Build history of the part. All positions in model axes, mm. Face numbers are marked on the shaded views. A direction names the side the tool comes from. Give positions to 0.01 mm unless a question says otherwise; leave off trailing zeros. Order: outer loops, then holes, each group sorted by start corner. A loop starts at its lowest first (then second) coordinate and runs counter-clockwise, first axis right, second up. Notation, with made-up numbers: (34.5, 33) -> (84.5, 33) arc R21 ccw to (84.5, 52) -> close; hole circle Ø3 at (89, 40.25). An arc over 180 degrees is marked (long way). One line per question, with ' | ' between items. Start each with the question number.
(1) Cut at C-C (z = 2.5). Give the cut face in (x, y), then the cut area to 3 significant figures.
(2) Pull direction X, two halves, no side cores. Call the marked faces 3, 4 and 5: +X half, -X half, draft (parallel to the pull), parting line (faces both ways), or undercut.
(3) Cut at B-B (x = -77). Give the cut face in (y, z).
(4) Which spindle directions (+Z, -Z, +X, -X, +Y, -Y) get a long thin tool onto all of the face, cutting with end or side? Do the marked faces 1 and 2. Say none if no direction does.
(5) Drill centre lines: L1, parallel to X at y = 14, z = 0.5; L2, parallel to Z at x = 1.3, y = 10; L3, parallel to Y at x = -2, z = -14.5. Where is each one in solid material? Low to high. Write a range as from..to.
(6) Cut at A-A (y = -12). Give the cut face in (x, z), then the cut area to 3 significant figures.
(7) Pin check, flat tips, straight feed: pin 1 Ø0.6 at (x, y) = (-23.5, -24) entering from +Z; pin 2 Ø3.5 at (x, y) = (-73.5, 20.5) entering from +Z. Stop position of each tip, or through.
(8) Cut at D-D (y = 10). Give the cut face in (x, z).
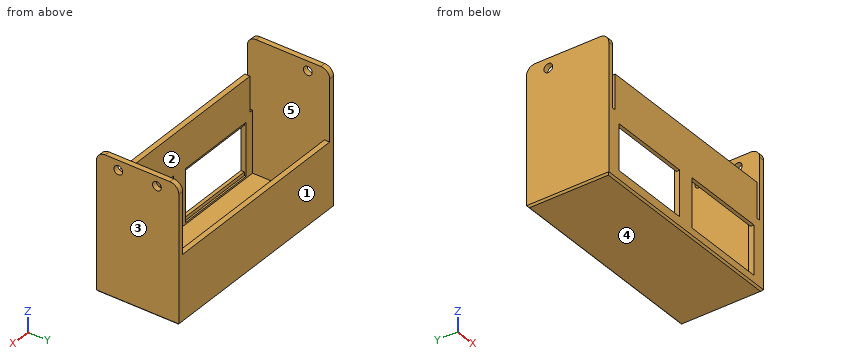
from build123d import *

# Parameters (mm, degrees)
F2_R      = 2.5
F3_DEPTH  = 3
F4_W      = 3
F4_H      = 35
F4_H_2    = 3
F4_W_2    = 41
F5_DEPTH  = 114
F6_R      = 2.5
F7_DEPTH  = 3
F8_W      = 110
F8_H      = 20
F9_DEPTH  = 3
F10_W     = 47
F10_H     = 26
F10_W_2   = 48
F10_H_2   = 28
F11_DEPTH = 3
F12_SIZE  = 1
F14_W     = 48
F14_H     = 2
F14_W_2   = 47
F15_DEPTH = 1


with BuildPart() as f3:
    # F2 (on Right) → F3 (new body)
    with BuildSketch(Plane.YZ):
        with BuildLine():
            ThreePointArc((22.5, 35), (21.0355339059, 38.5355339059), (17.5, 40))
            Line((17.5, 40), (-19.5, 40))
            ThreePointArc((-19.5, 40), (-23.0355339059, 38.5355339059), (-24.5, 35))
            Line((-24.5, 35), (-24.5, -38))
            Line((-24.5, -38), (22.5, -38))
            Line((22.5, -38), (22.5, 35))
        make_face()
        with Locations((-12, 34.5)):
            Circle(F2_R, mode=Mode.SUBTRACT)
        with Locations((10, 34.5)):
            Circle(F2_R, mode=Mode.SUBTRACT)
    extrude(amount=F3_DEPTH)

    # F4 (on Right) → F5 (join)
    with BuildSketch(Plane.YZ):
        with Locations((-23, -17.5)):
            Rectangle(F4_W, F4_H)
        with Locations((21, -36.5)):
            Rectangle(F4_W, F4_H_2)
        with Locations((21, -17.5)):
            Rectangle(F4_W, F4_H)
        with Locations((-1, -36.5)):
            Rectangle(F4_W_2, F4_H_2)
        with Locations((-23, -36.5)):
            Rectangle(F4_W, F4_H_2)
    extrude(amount=-F5_DEPTH)

    # F6 (on face) → F7 (join)
    with BuildSketch(Plane(origin=(-114, 0, 0), x_dir=(0, -1, 0), z_dir=(-1, 0, 0))):
        with BuildLine():
            ThreePointArc((24.5, 35), (23.0355339059, 38.5355339059), (19.5, 40))
            Line((19.5, 40), (-17.5, 40))
            ThreePointArc((-17.5, 40), (-21.0355339059, 38.5355339059), (-22.5, 35))
            Line((-22.5, 35), (-22.5, -38))
            Line((-22.5, -38), (24.5, -38))
            Line((24.5, -38), (24.5, 35))
        make_face()
        with Locations((-10, 34.5)):
            Circle(F6_R, mode=Mode.SUBTRACT)
    extrude(amount=F7_DEPTH)

    # F8 (on face) → F9 (join)
    with BuildSketch(Plane.XZ.offset(24.5)):
        with Locations((-57, 10)):
            Rectangle(F8_W, F8_H)
    extrude(amount=-F9_DEPTH)

    # F10 (on face) → F11 (cut, through all)
    with BuildSketch(Plane.XZ.offset(24.5)):
        with Locations((-85.5, -19)):
            Rectangle(F10_W, F10_H)
        with Locations((-28.5, -19)):
            Rectangle(F10_W_2, F10_H_2)
    extrude(amount=-F11_DEPTH, mode=Mode.SUBTRACT)

    # F12
    f12_edges = [f3.edges().sort_by_distance(p)[0] for p in [
        (-57, -24.5, -38),
        (3, -1, -38),
        (-57, 22.5, -38),
        (-117, -1, -38),
    ]]
    chamfer(f12_edges, length=F12_SIZE)

    # F14 (on face) → F15 (cut)
    with BuildSketch(Plane(origin=(0, -21.5, 0), x_dir=(-1, 0, 0), z_dir=(0, 1, 0))):
        with Locations((28.5, -34)):
            Rectangle(F14_W, F14_H)
        with Locations((85.5, -33)):
            Rectangle(F14_W_2, F14_H)
        with Locations((85.5, -5)):
            Rectangle(F14_W_2, F14_H)
        with Locations((28.5, -4)):
            Rectangle(F14_W, F14_H)
    extrude(amount=-F15_DEPTH, mode=Mode.SUBTRACT)


solid = f3.part
Result set:
1) outline: (-117, -24.5) -> (-114, -24.5) -> (-114, 22.5) -> (-117, 22.5) -> close; (-112, -24.5) -> (-2, -24.5) -> (-2, -21.5) -> (-112, -21.5) -> close; (0, -24.5) -> (3, -24.5) -> (3, 22.5) -> (0, 22.5) -> close | area: 612 mm2
2) face 3: +X half | face 4: draft | face 5: undercut
3) outline: (-24.5, -37) -> (-23.5, -38) -> (21.5, -38) -> (22.5, -37) -> (22.5, 0) -> (19.5, 0) -> (19.5, -35) -> (-21.5, -35) -> (-21.5, -34) -> (-22.5, -34) -> (-22.5, -32) -> (-24.5, -32) -> close; (-24.5, -6) -> (-22.5, -6) -> (-22.5, -4) -> (-21.5, -4) -> (-21.5, 20) -> (-24.5, 20) -> close
4) face 1: +Z, -Z, +X, -X, +Y | face 2: +Z
5) L1: x = -117..-114, 0..3 | L2: z = -38..32, 37..40 | L3: y = -24.5..-21.5, 19.5..22.5
6) outline: (-117, -37) -> (-116, -38) -> (2, -38) -> (3, -37) -> (3, 32) -> (0, 32) -> (0, -35) -> (-114, -35) -> (-114, 40) -> (-117, 40) -> close; (0, 37) -> (3, 37) -> (3, 40) -> (0, 40) -> close | area: 794 mm2
7) pin 1: stops at z = 20 | pin 2: stops at z = 0
8) outline: (-117, -37) -> (-116, -38) -> (2, -38) -> (3, -37) -> (3, 32) -> (0, 32) -> (0, -35) -> (-114, -35) -> (-114, 32) -> (-117, 32) -> close; (-117, 37) -> (-114, 37) -> (-114, 40) -> (-117, 40) -> close; (0, 37) -> (3, 37) -> (3, 40) -> (0, 40) -> close
